The model under review builds one solid part; all positions refer to its coordinate system, in mm. A direction names the side the tool comes from. Round coordinates to 2 decimals unless told otherwise and drop trailing zeros. Write each loop counter-clockwise with the first axis right and the second up, starting at its lowest first coordinate (ties: lowest second). Pieces come first, ordered by that corner, then holes. Notation, with made-up numbers: M 45.5,-26.5 L 57.5,-26.5 A20 cw 57.5,-14.5 Z; hole C 61.25,40 d5. An arc over 180 degrees is marked long. Write item = value, one per line. Start each with the question number.
Item 1: Take a section at C-C, the plane y = 0. Give the boundary of the cut face in (x, z) (3 decimals).
Item 2: Tool access review of faces 1 (the cylindrical face through (28.808, -0.028, -0.335)), 2 (the flat face through (1, -3, -1.5)), 3 (the flat face through (1, 4, 0)), 4 (the flat face through (2, 3, 1.5)), 5 (the flat face through (-23, 0, 0)): name each direction out of +Z, -Z, +X, -X, +Y, -Y from which nothing blocks a thin tool from reaching the whole face with its end or side.
Item 3: Take a section at B-B, the plane x = -14. Give the boundary of the cut face in (y, z), plus the area to 3 significant figures.
Item 4: For pin 1 Ø0.6 at (x, y) = (10, -3) entering from -Z; pin 2 Ø1 at (y, z) = (0, 1) entering from +X; pin 3 Ø3 at (x, y) = (-15, 1) entering from +Z, all flat-tipped, find the tip position at first contact; note any pin that passes through.
Item 5: The part is to be moulded in two halves that separate along Y. For faces 6 (the flat face through (1, -4, 0)), 7 (the cylindrical face through (-24.192, 0.056, -0.335)), 8 (the flat face through (3, 2, 0)), say which applies: +Y half, -Y half, draft (parallel to the pull), parting line (faces both ways), or undercut.
Item 6: Take a section at A-A, the plane z = 0. Give the boundary of the cut face in (x, y) (3 decimals).
Item 7: To check wall thickness, follow line 1 along X through (y, z) = (-1.5, -0.05); line 2 along Y through (x, z) = (9, -0.2); line 3 along Z through (x, y) = (-25, 2) (3 decimals). State the ranges of each line that lie inside material, in increasing order.
Item 8: Take a section at D-D, the plane y = 2.75. Give the boundary of the cut face in (x, z) (3 decimals).
from build123d import *

# Parameters (mm, degrees)
F0_R     = 0.875
F1_DEPTH = 4
F3_DEPTH = 2
F4_DEPTH = 4
F5_W     = 49
F5_H     = 4
F6_DEPTH = 2.5


with BuildPart() as f1:
    # F0 (on Front) → F1 (new body, symmetric)
    with BuildSketch(Plane.XZ):
        with BuildLine():
            ThreePointArc((-23, 1.5), (-27.5, 0), (-23, -1.5))
            Line((-23, -1.5), (26, -1.5))
            ThreePointArc((26, -1.5), (30.5, 0), (26, 1.5))
            Line((26, 1.5), (-23, 1.5))
        make_face()
        with Locations((-25, 0)):
            Circle(F0_R, mode=Mode.SUBTRACT)
        with Locations((28, 0)):
            Circle(F0_R, mode=Mode.SUBTRACT)
    extrude(amount=F1_DEPTH, both=True)

    # F2 (on Front) → F3 (cut, symmetric)
    with BuildSketch(Plane.XZ):
        with BuildLine():
            ThreePointArc((26, -1.5), (28.790569, -2.371708), (30.5, 0))
            ThreePointArc((30.5, 0), (28.790569, 2.371708), (26, 1.5))
            ThreePointArc((26, 1.5), (25.5, 0), (26, -1.5))
        make_face()
    extrude(amount=F3_DEPTH, both=True, mode=Mode.SUBTRACT)

    # F0 (on Front) → F4 (join, symmetric)
    with BuildSketch(Plane.XZ):
        with Locations((28, 0)):
            Circle(F0_R)
    extrude(amount=F4_DEPTH, both=True)

    # F5 (on Top) → F6 (cut, symmetric)
    with BuildSketch(Plane.XY):
        with Locations((1.5, 0)):
            Rectangle(F5_W, F5_H)
    extrude(amount=F6_DEPTH, both=True, mode=Mode.SUBTRACT)


solid = f1.part
Response values:
q1.outline = M -23,-1.5 L -23,1.5 A2.5 ccw long Z; C 28,0 d1.75; hole C -25,0 d1.75
q2.face_1 = none
q2.face_2 = -Z, +Y, -Y
q2.face_3 = +Z, -Z, +X, -X, +Y
q2.face_4 = +Z, +Y, -Y
q2.face_5 = +Z, -Z
q3.outline = M -4,-1.5 L -2,-1.5 L -2,1.5 L -4,1.5 Z; M 2,-1.5 L 4,-1.5 L 4,1.5 L 2,1.5 Z
q3.area = 12.0 mm2
q4.pin_1 = -1.5
q4.pin_2 = 28.72
q4.pin_3 = 1.5
q5.face_6 = -Y half
q5.face_7 = draft
q5.face_8 = undercut
q6.outline = M -27.5,-4 L -25.875,-4 L -25.875,4 L -27.5,4 Z; M -24.125,-4 L 30.5,-4 L 30.5,-2 L 28.875,-2 L 28.875,2 L 30.5,2 L 30.5,4 L -24.125,4 Z; hole M -23,-2 L 27.125,-2 L 27.125,2 L -23,2 Z
q7.line_1 = -27.5 to -25.87, -24.13 to -23, 27.13 to 28.87
q7.line_2 = -4 to -2, 2 to 4
q7.line_3 = -2.5 to -0.875, 0.875 to 2.5
q8.outline = M -23,-1.5 L 26,-1.5 A2.5 ccw long 26,1.5 L -23,1.5 A2.5 ccw long Z; hole C -25,0 d1.75
